The model under review builds one solid part; all positions refer to its coordinate system, in mm. A direction names the side the tool comes from. Round coordinates to 2 decimals unless told otherwise and drop trailing zeros. Loops run counter-clockwise (first coordinate to the right, second up) from the corner with the lowest first, then second, coordinate; pieces in that order, holes last. Notation, with made-up numbers: (-25, 66) -> (-10, 66) arc R16 ccw to (-10, 72) -> close; hole circle Ø11 at (-38, 38). An arc over 180 degrees is marked (long way). Use a Markdown table: item, result. Add a question column.
1) For faces 4 (the cylindrical face through (-315.036, -55.832, 8.874)), 5 (the flat face through (-10, 332, 0)), list the 3-axis set-ups (+Z, -Z, +X, -X, +Y, -Y) from which the entire face can be reached by the end or side of a thin tool; tool diameter is ignored.
2) Consider section D-D on y = 511.5. Give the boundary of the cut face in (x, z), plus the area to 3 significant figures.
3) Wall thickness on probe 1 along X at (y, z) = (-29, 6.75); probe 2 along X at (y, z) = (35, 10.25); probe 3 along Y at (x, z) = (-13, 9): over which ranges is each line inside the solid? List them lowest first.
4) Insertion check: pin 1 (5.5 mm diameter, centred on x = -469, z = 10.5, fed in from -Y); pin 2 (1.5 mm diameter, centred on x = -227, z = 8, fed in from +Y); pin 3 (9 mm diameter, centred on y = 129, z = 7.5, fed in from +X). Each pin has a flat end and moves straight along its axis. Give the tip position at first contact, or say it passes through.
5) Consider section B-B on z = 13.5. Give the boundary of the cut face in (x, y).
6) Mouldability with a two-part tool opening along X and no side actions: class faces 1 (the flat face through (-10, 332, 18)), 2 (the cylindrical face through (146.76, 719.28, 8.87)), 3 (the cylindrical face through (-285.742, 284.964, 8.874)) as released by +X, released by -X, zero draft, split by the parting line, or undercut.
7) Consider section A-A on y = 0. Give the boundary of the cut face in (x, z).
8) Consider section C-C on x = 0. Give the boundary of the cut face in (y, z).
from build123d import *

# Parameters (mm, degrees)
F1_DEPTH = 18


with BuildPart() as f1:
    # F0 (on Top) → F1 (new body)
    with BuildSketch(Plane.XY):
        with BuildLine():
            ThreePointArc((-300, 250), (-285.355339, 285.355339), (-250, 300))
            Line((-250, 300), (250, 300))
            ThreePointArc((250, 300), (285.355339, 285.355339), (300, 250))
            Line((300, 250), (300, -300))
            Line((300, -300), (300, -318))
            Line((300, -318), (661.646431, -318))
            ThreePointArc((661.646431, -318), (665.88404, -309.028228), (670, -300))
            ThreePointArc((670, -300), (128.426587, 722.777014), (-732.336483, -50.825933))
            ThreePointArc((-732.336483, -50.825933), (-731.603853, -60.463233), (-730.744404, -70.090053))
            Line((-730.744404, -70.090053), (-350, -70.090053))
            ThreePointArc((-350, -70.090053), (-314.644661, -55.445392), (-300, -20.090053))
            Line((-300, -20.090053), (-300, -2.090053))
            Line((-300, -2.090053), (-300, 250))
        make_face()
    extrude(amount=F1_DEPTH)


solid = f1.part
Result set:
| question | item | result |
|---|---|---|
| 1 | face 4 | +Z, -Z, -Y |
| 1 | face 5 | -Z, +X, -X, +Y, -Y |
| 2 | outline | (-526.56, 0) -> (526.56, 0) -> (526.56, 18) -> (-526.56, 18) -> close |
| 2 | area | 19,000 mm2 |
| 3 | probe 1 | -733.53 to -300.8, 300 to 733.53 |
| 3 | probe 2 | -733.26 to -300, 300 to 733.26 |
| 3 | probe 3 | 300 to 733.98 |
| 4 | pin 1 | y = -70.09 |
| 4 | pin 2 | y = 698.36 |
| 4 | pin 3 | x = 723.46 |
| 5 | outline | (-732.34, -50.83) arc R734.09 ccw to (-730.74, -70.09) -> (-350, -70.09) arc R50 ccw to (-300, -20.09) -> (-300, 250) arc R50 cw to (-250, 300) -> (250, 300) arc R50 cw to (300, 250) -> (300, -318) -> (661.65, -318) arc R734.09 ccw to (670, -300) arc R734.1 ccw (long way) to start |
| 6 | face 1 | zero draft |
| 6 | face 2 | split by the parting line |
| 6 | face 3 | undercut |
| 7 | outline | (-734.1, 0) -> (-300, 0) -> (-300, 18) -> (-734.1, 18) -> close; (300, 0) -> (734.1, 0) -> (734.1, 18) -> (300, 18) -> close |
| 8 | outline | (300, 0) -> (734.1, 0) -> (734.1, 18) -> (300, 18) -> close |
